from build123d import *

# Parameters (mm, degrees)
SKETCH1_W           = 54.585576923
SKETCH1_H           = 4.7625
SKETCH1_W_2         = 4.7625
SKETCH1_W_3         = 59.348076923
SKETCH1_H_2         = 26.760714285
SKETCH1_H_3         = 26.760714286
BOSS_EXTRUDE1_DEPTH = 4.7625
SKETCH2_W           = 4.7625
SKETCH2_H           = 12.7
CUT_EXTRUDE1_DEPTH  = 397.998805689


with BuildPart() as part:
    # Sketch1 → Boss-Extrude1 (new body)
    with BuildSketch(Plane(origin=(0, 0, 0), x_dir=(1, 0, 0), z_dir=(0, 1, 0))):
        Polygon((0, -88.9), (0, 88.9), (-29.674038462, 88.9), (-89.022115385, 88.9), (-148.370192308, 88.9), (-207.718269231, 88.9), (-267.066346154, 88.9), (-326.414423077, 88.9), (-381, 88.9), (-381, 66.901785714), (-381, 40.141071429), (-381, 13.380357143), (-381, -13.380357143), (-381, -40.141071429), (-381, -66.901785714), (-381, -88.9), (-326.414423077, -88.9), (-267.066346154, -88.9), (-207.718269231, -88.9), (-148.370192308, -88.9), (-89.022115385, -88.9), (-29.674038462, -88.9), align=None)
        Polygon((29.674038462, 88.9), (0, 88.9), (0, -88.9), (29.674038462, -88.9), (89.022115385, -88.9), (148.370192308, -88.9), (207.718269231, -88.9), (267.066346154, -88.9), (326.414423077, -88.9), (381, -88.9), (381, -66.901785714), (381, -40.141071429), (381, -13.380357143), (381, 13.380357143), (381, 40.141071429), (381, 66.901785714), (381, 88.9), (326.414423077, 88.9), (267.066346154, 88.9), (207.718269231, 88.9), (148.370192308, 88.9), (89.022115385, 88.9), align=None)
        with Locations((-353.707211539, -91.28125)):
            Rectangle(SKETCH1_W, SKETCH1_H)
        with Locations((-383.38125, -91.28125)):
            Rectangle(SKETCH1_W_2, SKETCH1_H)
        with Locations((-237.392307693, -91.28125)):
            Rectangle(SKETCH1_W_3, SKETCH1_H)
        with Locations((-383.38125, -53.521428571)):
            Rectangle(SKETCH1_W_2, SKETCH1_H_2)
        with Locations((-118.696153847, -91.28125)):
            Rectangle(SKETCH1_W_3, SKETCH1_H)
        with Locations((-383.38125, 0)):
            Rectangle(SKETCH1_W_2, SKETCH1_H_3)
        with Locations((-383.38125, 53.521428571)):
            Rectangle(SKETCH1_W_2, SKETCH1_H_2)
        with Locations((-383.38125, 91.28125)):
            Rectangle(SKETCH1_W_2, SKETCH1_H)
        with Locations((-353.707211539, 91.28125)):
            Rectangle(SKETCH1_W, SKETCH1_H)
        with Locations((-237.392307693, 91.28125)):
            Rectangle(SKETCH1_W_3, SKETCH1_H)
        with Locations((-118.696153847, 91.28125)):
            Rectangle(SKETCH1_W_3, SKETCH1_H)
        Polygon((-29.674038462, 88.9), (0, 88.9), (29.674038462, 88.9), (29.674038462, 93.6625), (-29.674038462, 93.6625), align=None)
        with Locations((118.696153847, 91.28125)):
            Rectangle(SKETCH1_W_3, SKETCH1_H)
        Polygon((29.674038462, -88.9), (0, -88.9), (-29.674038462, -88.9), (-29.674038462, -93.6625), (29.674038462, -93.6625), align=None)
        with Locations((118.696153847, -91.28125)):
            Rectangle(SKETCH1_W_3, SKETCH1_H)
        with Locations((237.392307693, -91.28125)):
            Rectangle(SKETCH1_W_3, SKETCH1_H)
        with Locations((237.392307693, 91.28125)):
            Rectangle(SKETCH1_W_3, SKETCH1_H)
        with Locations((383.38125, 91.28125)):
            Rectangle(SKETCH1_W_2, SKETCH1_H)
        with Locations((383.38125, 53.521428571)):
            Rectangle(SKETCH1_W_2, SKETCH1_H_2)
        with Locations((383.38125, 0)):
            Rectangle(SKETCH1_W_2, SKETCH1_H_3)
        with Locations((383.38125, -53.521428571)):
            Rectangle(SKETCH1_W_2, SKETCH1_H_2)
        with Locations((383.38125, -91.28125)):
            Rectangle(SKETCH1_W_2, SKETCH1_H)
        with Locations((356.088461539, -91.28125)):
            Rectangle(SKETCH1_W_3, SKETCH1_H)
        with Locations((356.088461539, 91.28125)):
            Rectangle(SKETCH1_W_3, SKETCH1_H)
    extrude(amount=BOSS_EXTRUDE1_DEPTH)

    # Sketch2 → Cut-Extrude1 (cut, through all)
    with BuildSketch(Plane(origin=(0, 4.7625, 0), x_dir=(1, 0, 0), z_dir=(0, 1, 0))):
        with Locations((-121.44375, 82.55)):
            Rectangle(SKETCH2_W, SKETCH2_H)
        with Locations((-121.44375, -82.55)):
            Rectangle(SKETCH2_W, SKETCH2_H)
        with Locations((132.55625, 82.55)):
            Rectangle(SKETCH2_W, SKETCH2_H)
        with Locations((132.55625, -82.55)):
            Rectangle(SKETCH2_W, SKETCH2_H)
    extrude(amount=-CUT_EXTRUDE1_DEPTH, mode=Mode.SUBTRACT)


solid = part.part
Work out the finished part from the listing and answer in its coordinate system (mm). Coordinates: 2 decimals unless noted, no trailing zeros. Loops run counter-clockwise (first coordinate to the right, second up) from the corner with the lowest first, then second, coordinate; pieces in that order, holes last. Notation, with made-up numbers: (31, 73) -> (76, 73) arc R36 ccw to (76, 107) -> close; hole circle Ø2 at (35.5, 29). An arc over 180 degrees is marked (long way). Answer as CSV lines item,"result".
1) The part is cut by section A-A (y = 3.65). State how many separate pieces and enclosed holes the cut face has, and give its area (3 significant figures).
A:
separate pieces,"1"
enclosed holes,"4"
area,"140,000 mm²"
2) Flat-ended cylindrical pins translate along their axes: pin 1 (1.4 mm diameter, centred on x = -58.5, y = 2, fed in from -Z); pin 2 (1.5 mm diameter, centred on y = 1, z = 34.5, fed in from +X); pin 3 (1.4 mm diameter, centred on y = 3, z = 83, fed in from -X). Find the tip coordinate at first contact, or state that the pin passes through.
A:
pin 1,"stops at z = -88.9"
pin 2,"stops at x = 381"
pin 3,"stops at x = -381"
3) Straight lines are drawn through the part: probe 1 along X at (y, z) = (3.7, 81.5) (1 decimal); probe 2 along Z at (x, y) = (134, 2.2); probe 3 along Z at (x, y) = (-152, 4.15). For each, find the intervals that lie inside material, in ascending order.
A:
probe 1,"x = -381 to -123.8, -119.1 to 130.2, 134.9 to 381"
probe 2,"z = -93.66 to -88.9, -76.2 to 76.2, 88.9 to 93.66"
probe 3,"z = -88.9 to 88.9"
4) The part is cut by section B-B (x = 66). Give the vertices of the cut face in (y, z).
A:
outline,"(0, -88.9) -> (4.76, -88.9) -> (4.76, 88.9) -> (0, 88.9) -> close"
